Drawing for the job (mm, zero at the part's lowest x, y, z). A direction names the side the tool comes from. Round coordinates to 2 decimals unless told otherwise and drop trailing zeros. Loops run counter-clockwise (first coordinate to the right, second up) from the corner with the lowest first, then second, coordinate; pieces in that order, holes last. Notation, with made-up numbers: M 21,31 L 74,31 A8 ccw 74,45 Z; hole C 1.5,-20 d5. An arc over 180 degrees is marked long. Write each question's results on one line, items separated by ' | '.
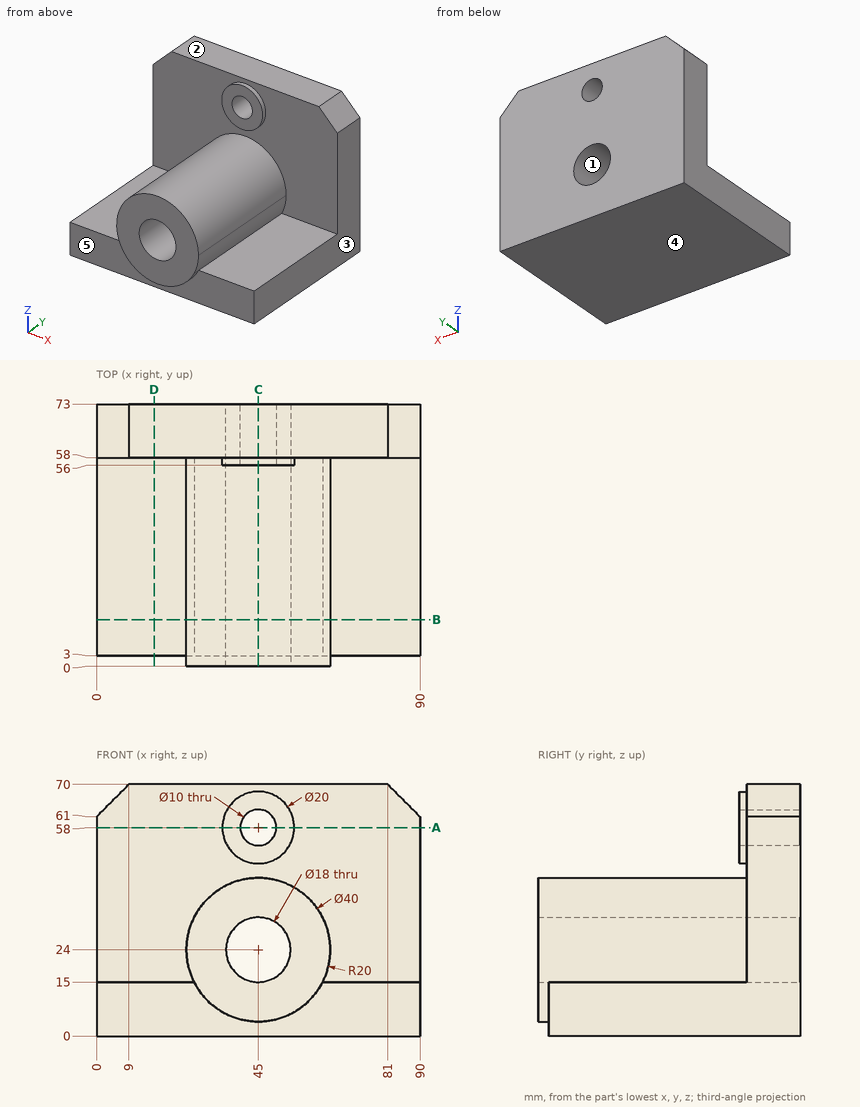
Item 1: Band-saw the part on C-C on x = 45. Give the cut face in (y, z), and give its area (3 significant figures).
Filled sheet:
outline: M 0,4 L 3,4 L 3,0 L 73,0 L 73,15 L 0,15 Z; M 0,33 L 73,33 L 73,53 L 56,53 L 56,48 L 58,48 L 58,44 L 0,44 Z; M 56,63 L 73,63 L 73,70 L 58,70 L 58,68 L 56,68 Z | area: 2,150 mm^2
Item 2: Drop flat-ended pins along their axis: P1, Ø16.5, axis at x = 39.5, z = 37.5, coming from the -Y side; P2, Ø22, axis at x = 43.5, z = 61.5, coming from the -Y side; P3, Ø1, axis at x = 41, z = 18, coming from the +Y side; P4, Ø8, axis at x = 11, y = 21, coming from the +Z side. Give the stop position or say it passes through.
Filled sheet:
P1: y = 0 | P2: y = 56 | P3: through | P4: z = 15
Item 3: Band-saw the part on B-B on y = 13. Give the cut face in (x, z), and give its area (3 significant figures).
Filled sheet:
outline: M 0,0 L 90,0 L 90,15 L 62.86,15 A20 ccw 65,24 A20 ccw long 27.14,15 L 0,15 Z; hole C 45,24 d18 | area: 2,070 mm^2
Item 4: Which spindle directions (+Z, -Z, +X, -X, +Y, -Y) get a long thin tool onto all of the face, cutting with end or side? Do the marked faces 4 and 5. Say none if no direction does.
Filled sheet:
face 4: -Z, +X, -X, +Y, -Y | face 5: -Z, -Y
Item 5: Band-saw the part on A-A on z = 58. Give the cut face in (x, y).
Filled sheet:
outline: M 0,58 L 35,58 L 35,56 L 40,56 L 40,73 L 0,73 Z; M 50,56 L 55,56 L 55,58 L 90,58 L 90,73 L 50,73 Z
Item 6: Band-saw the part on D-D on x = 16. Give the cut face in (y, z), and give its area (4 significant figures).
Filled sheet:
outline: M 3,0 L 73,0 L 73,70 L 58,70 L 58,15 L 3,15 Z | area: 1,875 mm^2
Item 7: Wall check: L1, parallel to Z at x = 45, y = 65.75; L2, parallel to Z at x = 45, y = 21; L3, parallel to Y at x = 85, z = 8. Give the ranges that are in metal, low to high.
Filled sheet:
L1: 0 to 15, 33 to 53, 63 to 70 | L2: 0 to 15, 33 to 44 | L3: 3 to 73
Item 8: Two-plate mould, pull along X, no slides. Class the marked faces 1, 2 and 3: +X half, -X half, draft (parallel to the pull), parting line (faces both ways), or undercut.
Filled sheet:
face 1: undercut | face 2: draft | face 3: +X half
